Read the model definition and answer for the solid it produces. Units are mm, in the model's axes. A direction names the side the tool comes from. Coordinates: 2 decimals unless noted, no trailing zeros. Loops run counter-clockwise (first coordinate to the right, second up) from the corner with the lowest first, then second, coordinate; pieces in that order, holes last.
from build123d import *

# Parameters (mm, degrees)
SKETCH1_W           = 320
SKETCH1_H           = 370
BOSS_EXTRUDE1_DEPTH = 3
SKETCH2_W           = 280
SKETCH2_H           = 310
SKETCH2_W_2         = 275
SKETCH2_H_2         = 304.464285714
BOSS_EXTRUDE2_DEPTH = 65
SKETCH4_W           = 15
SKETCH4_H           = 175
CUT_EXTRUDE2_DEPTH  = 40
SKETCH5_R           = 3.5
CUT_EXTRUDE3_DEPTH  = 359.955428988
SKETCH6_W           = 38
SKETCH6_H           = 38
CUT_EXTRUDE5_DEPTH  = 2


with BuildPart() as part:
    # Sketch1 → Boss-Extrude1 (new body)
    with BuildSketch(Plane(origin=(0, 0, 0), x_dir=(1, 0, 0), z_dir=(0, 1, 0))):
        Rectangle(SKETCH1_W, SKETCH1_H)
    extrude(amount=BOSS_EXTRUDE1_DEPTH)

    # Sketch2 → Boss-Extrude2 (add)
    with BuildSketch(Plane(origin=(0, 3, 0), x_dir=(1, 0, 0), z_dir=(0, 1, 0))):
        Rectangle(SKETCH2_W, SKETCH2_H)
        Rectangle(SKETCH2_W_2, SKETCH2_H_2, mode=Mode.SUBTRACT)
    extrude(amount=BOSS_EXTRUDE2_DEPTH)

    # Sketch4 → Cut-Extrude2 (cut)
    with BuildSketch(Plane(origin=(0, 3, 0), x_dir=(1, 0, 0), z_dir=(0, 1, 0))):
        with Locations((-152.5, -77.5)):
            Rectangle(SKETCH4_W, SKETCH4_H)
    cut_extrude2 = extrude(amount=-CUT_EXTRUDE2_DEPTH, mode=Mode.SUBTRACT)

    # Mirror3: Cut-Extrude2 across plane
    add(cut_extrude2.mirror(Plane(origin=(0, 0, 0), x_dir=(0, 0, 1), z_dir=(1, 0, 0))), mode=Mode.SUBTRACT)

    # Sketch5 → Cut-Extrude3 (cut, through all)
    with BuildSketch(Plane(origin=(140, 0, 0), x_dir=(0, 0, -1), z_dir=(1, 0, 0))):
        with Locations((-77.5, 23)):
            Circle(SKETCH5_R)
    extrude(amount=-CUT_EXTRUDE3_DEPTH, mode=Mode.SUBTRACT)

    # Sketch6 → Cut-Extrude5 (cut)
    with BuildSketch(Plane.XZ):
        with Locations((-81, -116)):
            Rectangle(SKETCH6_W, SKETCH6_H)
        with Locations((81, -116)):
            Rectangle(SKETCH6_W, SKETCH6_H)
    extrude(amount=-CUT_EXTRUDE5_DEPTH, mode=Mode.SUBTRACT)


solid = part.part
Q1. A cutting plane is placed at A-A (y = 34). Give the vertices of the cut face in (x, z).
Findings below:
outline: (-140, -155) - (140, -155) - (140, 155) - (-140, 155) - close; hole (-137.5, -152.23) - (137.5, -152.23) - (137.5, 152.23) - (-137.5, 152.23) - close
Q2. A cutting plane is placed at C-C (z = -103.5). Give the vertices of the cut face in (x, y).
Findings below:
outline: (-160, 0) - (-100, 0) - (-100, 2) - (-62, 2) - (-62, 0) - (62, 0) - (62, 2) - (100, 2) - (100, 0) - (160, 0) - (160, 3) - (140, 3) - (140, 68) - (137.5, 68) - (137.5, 3) - (-137.5, 3) - (-137.5, 68) - (-140, 68) - (-140, 3) - (-160, 3) - close
Q3. Flat-ended cylindrical pins translate along their axes: pin 1 Ø3 at (y, z) = (36.5, 86.5) entering from +X; pin 2 Ø2 at (x, y) = (68, 41) entering from +Z; pin 3 Ø2 at (x, z) = (117.5, -6) entering from -Y; pin 4 Ø0.9 at (y, z) = (2, 80) entering from +X. Find the tip coordinate at first contact, or state that the pin passes through.
Findings below:
pin 1: stops at x = 140
pin 2: stops at z = 155
pin 3: stops at y = 0
pin 4: stops at x = 145
Q4. Determine the mould class of faces 1 (the face through (-2, 35, -155)), 2 (the face through (-140, 35, 2)), 3 (the face through (-2, 35, 152.232)), 4 (the face through (140, 35, 2)) for opening direction X: +X half, -X half, draft (parallel to the pull), parting line (faces both ways), or undercut.
Findings below:
face 1: draft
face 2: -X half
face 3: undercut
face 4: +X half
Q5. A cutting plane is placed at D-D (z = 28). Give the vertices of the cut face in (x, y), then the cut area to 4 significant figures.
Findings below:
outline: (-145, 0) - (145, 0) - (145, 3) - (140, 3) - (140, 68) - (137.5, 68) - (137.5, 3) - (-137.5, 3) - (-137.5, 68) - (-140, 68) - (-140, 3) - (-145, 3) - close
area: 1,195 mm2
Q6. Straight lines are drawn through the part: probe 1 along Z at (x, y) = (91.5, 33.5); probe 2 along X at (y, z) = (30.5, -49); probe 3 along Y at (x, z) = (139.25, 77.5). For each, find the intervals that lie inside material, in ascending order.
Findings below:
probe 1: z = -155 to -152.23, 152.23 to 155
probe 2: x = -140 to -137.5, 137.5 to 140
probe 3: y = 0 to 19.5, 26.5 to 68
Q7. Which of the six approach directions +Z, -Z, +X, -X, +Y, -Y give full straight-line access (tool end or side, diameter ignored) to faces 5 (the face through (-2, 35, 155)), 6 (the face through (-81, 2, -116)), 7 (the face through (-2, 0, -3)), 8 (the face through (-143, 3, -28))?
Findings below:
face 5: +Z, +X, -X, +Y
face 6: -Y
face 7: +Z, -Z, +X, -X, -Y
face 8: +Y
Q8. A cutting plane is placed at B-B (x = 16.5). Give the vertices of the cut face in (y, z).
Findings below:
outline: (0, -185) - (3, -185) - (3, -155) - (68, -155) - (68, -152.23) - (3, -152.23) - (3, 152.23) - (68, 152.23) - (68, 155) - (3, 155) - (3, 185) - (0, 185) - close
